Check sheet for the modelled part. Datum: model origin and axes. Units: mm. A direction names the side the tool comes from. Coordinates: 2 decimals unless noted, no trailing zeros. Loops run counter-clockwise (first coordinate to the right, second up) from the corner with the lowest first, then second, coordinate; pieces in that order, holes last. Notation, with made-up numbers: M -11,35 L 17,35 A32 cw 17,66 Z; hole C 48.25,-10 d8. An arc over 180 degrees is marked long. Answer as CSV lines item,"result". Start each with the question number.
from build123d import *

# Parameters (mm, degrees)
F0_R     = 2.38125
F1_DEPTH = 6.35
F2_R     = 1.5875
F3_DEPTH = 6.35
F4_W     = 4.7752
F4_H     = 4.7752
F4_R     = 2.38125
F5_DEPTH = 2.54
F6_DEPTH = 6.35


with BuildPart() as f1:
    # F0 (on Top) → F1 (new body)
    with BuildSketch(Plane.XY):
        Circle(F0_R)
    extrude(amount=F1_DEPTH)

    # F2 (on face) → F3 (cut)
    with BuildSketch(Plane.XY.offset(6.35)):
        Circle(F2_R)
    extrude(amount=-F3_DEPTH, mode=Mode.SUBTRACT)

    # F4 (on face) → F5 (join)
    with BuildSketch(Plane(origin=(0, 0, 0), x_dir=(1, 0, 0), z_dir=(0, 0, -1))):
        Rectangle(F4_W, F4_H)
        Circle(F4_R, mode=Mode.SUBTRACT)
    extrude(amount=-F5_DEPTH)

    # F6 (add): a face of the model
    f6_faces = [f1.faces().sort_by_distance(p)[0] for p in [
        (-2.320068474, 0, 0),
    ]]
    extrude(f6_faces, amount=F6_DEPTH)


solid = f1.part
Item 1: Material ranges on line 1 (Y direction, x = 0, z = -1.75); line 2 (X direction, y = -0.1, z = 2); line 3 (X direction, y = -1.2, z = 5.5), recorded low to high. Write a range as from..to.
Item 2: Release check for a two-part mould opening along Y. For faces 3 (the face through (-1.89, -1.45, 4.42)), 4 (the face through (-0.34, -1.55, 0.09)), 5 (the face through (2.388, 0, -2)), 6 (the face through (0, -2.388, -2)) record: released by +Y, released by -Y, zero draft, split by the parting line, or undercut.
Item 3: Sectioned sample at C-C, the plane z = -5. Record the boundary of the cut face in (x, y) (1 decimal), and give its area (3 significant figures).
Item 4: Set-up check for faces 1 (the face through (-2, -2, 2.54)), 2 (the face through (0, -2, -6.35)): record each of +Z, -Z, +X, -X, +Y, -Y from which the full face is reachable in a straight line by a thin tool's end or side.
Item 5: Sectioned sample at D-D, the plane y = -2. Record the boundary of the cut face in (x, z).
Reply:
1,line 1,"-2.39..-1.59, 1.59..2.39"
1,line 2,"-2.39..-1.58, 1.58..2.39"
1,line 3,"-2.06..-1.04, 1.04..2.06"
2,face 3,"split by the parting line"
2,face 4,"undercut"
2,face 5,"zero draft"
2,face 6,"released by -Y"
3,outline,"M -2.4,-2.4 L 2.4,-2.4 L 2.4,2.4 L -2.4,2.4 Z; hole C 0,0 d3.2"
3,area,"14.9 mm²"
4,face 1,"+Z"
4,face 2,"-Z, +X, -X, +Y, -Y"
5,outline,"M -2.39,-6.35 L 2.39,-6.35 L 2.39,2.54 L 1.29,2.54 L 1.29,6.35 L -1.29,6.35 L -1.29,2.54 L -2.39,2.54 Z"
